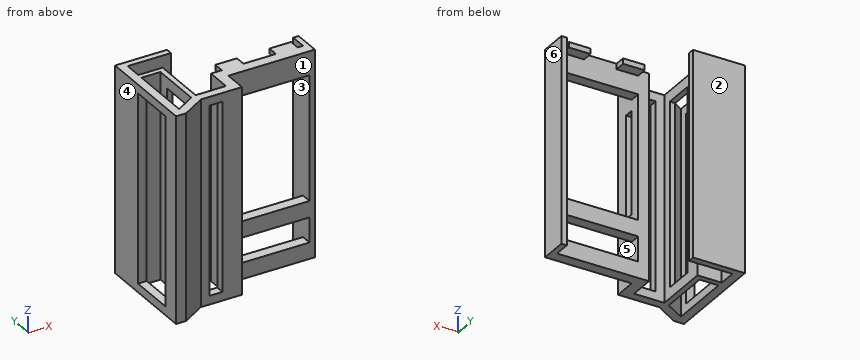
from build123d import *

# Parameters (mm, degrees)
EXTRUDE_1_DEPTH        = 190
CUT_EXTRUDE_1_DEPTH    = 235.752853891
SKETCH_4_W             = 75
SKETCH_4_H             = 23
CUT_EXTRUDE_2_DEPTH    = 230.181151057
SKETCH_6_W             = 75
SKETCH_6_H             = 115
CUT_EXTRUDE_3_DEPTH    = 230.181151057
SKETCH_7_W             = 20
SKETCH_7_H             = 5
EXTRUDE_3_DEPTH        = 10
PATTERN_LINEAR_1_COUNT = 2
PATTERN_LINEAR_1_PITCH = 50
CUT_EXTRUDE_4_REACH    = 220.14
SKETCH_8_W             = 95
SKETCH_8_H             = 8.95125425
CUT_EXTRUDE_5_REACH    = 237.272
SKETCH_9_W             = 12
SKETCH_9_H             = 174
CUT_EXTRUDE_6_REACH    = 239.306
SKETCH_10_W            = 170
SKETCH_10_H            = 27.319431914
CUT_EXTRUDE_7_REACH    = 248.83
SKETCH_12_W            = 174
SKETCH_12_H            = 41.774248955


with BuildPart() as part:
    # 草图1 → 凸台-拉伸1 (new body)
    with BuildSketch(Plane.XY):
        Polygon((0, 0), (-22.5, 0), (-22.5, 16.3), (17.5, 16.3), (17.5, 22.3), (-30.5, 22.3), (-30.5, -71.308501668), (-21.186581166, -71.308501668), (0, -58.65125425), (38, -58.65125425), (38, -37.7), (118, -37.7), (118, -12.7), (113, -12.7), (113, -27.7), (28, -27.7), (28, -50.7), (0, -50.7), align=None)
    extrude(amount=EXTRUDE_1_DEPTH)

    # 草图2 → 切除-拉伸1 (cut, through all)
    with BuildSketch(Plane.XY.offset(190)):
        Polygon((-22.5, -5), (-22.5, -62.774248955), (-5, -52.319431914), (-5, -5), align=None)
    extrude(amount=-CUT_EXTRUDE_1_DEPTH, mode=Mode.SUBTRACT)

    # 草图4 → 切除-拉伸2 (cut, through all)
    with BuildSketch(Plane(origin=(0, -27.7, 0), x_dir=(1, 0, 0), z_dir=(0, 1, 0))):
        with Locations((75.5, -26.5)):
            Rectangle(SKETCH_4_W, SKETCH_4_H)
    extrude(amount=-CUT_EXTRUDE_2_DEPTH, mode=Mode.SUBTRACT)

    # 草图6 → 切除-拉伸3 (cut, through all)
    with BuildSketch(Plane(origin=(0, -27.7, 0), x_dir=(1, 0, 0), z_dir=(0, 1, 0))):
        with Locations((75.5, -110.5)):
            Rectangle(SKETCH_6_W, SKETCH_6_H)
    extrude(amount=-CUT_EXTRUDE_3_DEPTH, mode=Mode.SUBTRACT)

    # 草图7 → 凸台-拉伸3 (add)
    with BuildSketch(Plane(origin=(0, -27.7, 0), x_dir=(1, 0, 0), z_dir=(0, 1, 0))):
        with Locations((48, -187.5)):
            Rectangle(SKETCH_7_W, SKETCH_7_H)
    extrude_3 = extrude(amount=EXTRUDE_3_DEPTH)

    # 阵列(线性)1: 凸台-拉伸3 ×2
    with Locations(*[(i * PATTERN_LINEAR_1_PITCH, 0, 0) for i in range(1, PATTERN_LINEAR_1_COUNT)]):
        add(extrude_3)

    # 草图8 → 切除-拉伸4 (cut, up to next)
    with BuildSketch(Plane(origin=(38, 0, 0), x_dir=(0, 0, -1), z_dir=(1, 0, 0)), mode=Mode.PRIVATE) as cut_extrude_4_sk1:
        with Locations((-110.5, -42.175627125)):
            Rectangle(SKETCH_8_W, SKETCH_8_H)
    cut_extrude_4_tool1 = extrude(cut_extrude_4_sk1.sketch, amount=-CUT_EXTRUDE_4_REACH, mode=Mode.PRIVATE) & part.part
    add(cut_extrude_4_tool1.solids().sort_by_distance((38, -42.175627, 110.5))[0], mode=Mode.SUBTRACT)

    # 草图9 → 切除-拉伸5 (cut, up to next)
    with BuildSketch(Plane(origin=(0, -50.7, 0), x_dir=(1, 0, 0), z_dir=(0, 1, 0)), mode=Mode.PRIVATE) as cut_extrude_5_sk1:
        with Locations((14, -95)):
            Rectangle(SKETCH_9_W, SKETCH_9_H)
    cut_extrude_5_tool1 = extrude(cut_extrude_5_sk1.sketch, amount=-CUT_EXTRUDE_5_REACH, mode=Mode.PRIVATE) & part.part
    add(cut_extrude_5_tool1.solids().sort_by_distance((14, -50.7, 95))[0], mode=Mode.SUBTRACT)

    # 草图10 → 切除-拉伸6 (cut, up to next)
    with BuildSketch(Plane.ZY.offset(5), mode=Mode.PRIVATE) as cut_extrude_6_sk1:
        with Locations((95, -28.659715957)):
            Rectangle(SKETCH_10_W, SKETCH_10_H)
    cut_extrude_6_tool1 = extrude(cut_extrude_6_sk1.sketch, amount=-CUT_EXTRUDE_6_REACH, mode=Mode.PRIVATE) & part.part
    add(cut_extrude_6_tool1.solids().sort_by_distance((-5, -28.659716, 95))[0], mode=Mode.SUBTRACT)

    # 草图12 → 切除-拉伸7 (cut, up to next)
    with BuildSketch(Plane(origin=(-22.5, 0, 0), x_dir=(0, 0, -1), z_dir=(1, 0, 0)), mode=Mode.PRIVATE) as cut_extrude_7_sk1:
        with Locations((-95, -33.887124478)):
            Rectangle(SKETCH_12_W, SKETCH_12_H)
    cut_extrude_7_tool1 = extrude(cut_extrude_7_sk1.sketch, amount=-CUT_EXTRUDE_7_REACH, mode=Mode.PRIVATE) & part.part
    add(cut_extrude_7_tool1.solids().sort_by_distance((-22.5, -33.887124, 95))[0], mode=Mode.SUBTRACT)


solid = part.part
Input: part model. Units: mm. Frame: model coordinates. Face numbers are marked on the shaded views. A direction names the side the tool comes from. Round coordinates to 2 decimals unless told otherwise and drop trailing zeros. Write each loop counter-clockwise with the first axis right and the second up, starting at its lowest first coordinate (ties: lowest second). Pieces come first, ordered by that corner, then holes.
1) Contact query for flat-ended pins moving along their axis: P1, Ø2, axis at y = -22, z = 162.5, coming from the -X side; P2, Ø4, axis at x = 115, z = 107, coming from the +Y side; P3, Ø8.5, axis at y = -55, z = 57, coming from the +X side; P4, Ø10, axis at x = 45, y = -50, coming from the +Z side. Output: stop coordinate, or through.
2) Cut plane A-A (y = -30.5). Return the cut outline in (x, z).
3) Cut plane C-C (z = 28). Count the separate pieces of the cut face and the enclosed holes in it, then the cut area to 3 significant figures.
4) Draft query along X for the marked faces 4, 5 and 6. Return one class per face: pulls with the +X half, pulls with the -X half, needs draft (parallel to the pull), parting line crosses it, or undercut.
5) Cut plane D-D (y = -8). Return the cut outline in (x, z).
6) Cut plane B-B (x = 83.5). Return the cut outline in (y, z), then the cut area to 3 significant figures.
7) Ray query, L1, parallel to Y at x = -20.5, z = 97; L2, parallel to X at y = -37, z = 73.5; L3, parallel to Y at x = -21.5, z = 59.5. Return the intervals inside material, ascending.
8) Reachability of the marked faces 1, 2 and 3 from +Z, -Z, +X, -X, +Y, -Y: full face, straight path, thin tool, end or side. Return the list, or none.
Geometry says:
1. P1: stops at x = 113
1. P2: stops at y = -12.7
1. P3: stops at x = 38
1. P4: passes through
2. outline: (-30.5, 0) - (-22.5, 0) - (-22.5, 8) - (-30.5, 8) - close; (-30.5, 182) - (-22.5, 182) - (-22.5, 190) - (-30.5, 190) - close; (-5, 0) - (0, 0) - (0, 10) - (-5, 10) - close; (-5, 180) - (0, 180) - (0, 190) - (-5, 190) - close; (28, 0) - (118, 0) - (118, 190) - (28, 190) - close; hole (38, 15) - (113, 15) - (113, 38) - (38, 38) - close; hole (38, 53) - (113, 53) - (113, 168) - (38, 168) - close
3. separate pieces: 4
3. enclosed holes: 0
3. area: 1,630 mm2
4. face 4: pulls with the -X half
4. face 5: undercut
4. face 6: pulls with the +X half
5. outline: (-30.5, 0) - (-22.5, 0) - (-22.5, 190) - (-30.5, 190) - close; (-5, 0) - (0, 0) - (0, 190) - (-5, 190) - close
6. outline: (-37.7, 0) - (-27.7, 0) - (-27.7, 15) - (-37.7, 15) - close; (-37.7, 38) - (-27.7, 38) - (-27.7, 53) - (-37.7, 53) - close; (-37.7, 168) - (-27.7, 168) - (-27.7, 190) - (-37.7, 190) - close
6. area: 520 mm2
7. L1: y = -70.9 to -61.58, -5 to 0, 16.3 to 22.3
7. L2: x = 28 to 38, 113 to 118
7. L3: y = -71.31 to -62.18, -5 to 0, 16.3 to 22.3
8. face 1: +Z, -Z, +X, -Y
8. face 2: +Z, -Z, +X, -X, +Y
8. face 3: +Y
